Autodesk Inventor part; units mm, degrees
ref_plane "YZ Plane" through (0, 0, 0) normal (1, 0, 0) x (0, 1, 0)
ref_plane "XZ Plane" through (0, 0, 0) normal (0, 1, 0) x (-1, 0, 0)
ref_plane "XY Plane" through (0, 0, 0) normal (0, 0, 1) x (1, 0, 0)
sketch "Sketch1" plane through (0, 0, 0) normal (0, 0, 1) x (1, 0, 0)
  line L0 (-94, 50) -> (94, 50)
  line L1 (94, 50) -> (94, -50)
  line L2 (94, -50) -> (-94, -50)
  line L3 (-94, -50) -> (-94, 50)
  point P0 (0, 0)
  point P1 (0, 50)
  point P2 (94, 0)
  dimension "d2" = 100
  dimension "d3" = 188
extrude "Extrusion1" add sketch "Sketch1" along normal blind 6
sketch "Sketch5" plane through (0, 0, 6) normal (0, 0, 1) x (1, 0, 0)
  circle A0 centre (82, -43.9615) radius 1.7
  circle A1 centre (82, 43.9615) radius 1.7
  line L0 (82, -43.9615) -> (82, 43.9615) construction
  line L1 (94, -50) -> (94, 50)
  point P0 (0, 0)
  point P1 (82, 0)
  point P2 (94, 0)
  dimension "d27" = 3.4
  dimension "d28" = 12
  dimension "d29" = 87.923
extrude "Extrusion5" cut sketch "Sketch5" against normal through all
sketch "Sketch6" plane through (0, 0, 6) normal (0, 0, 1) x (1, 0, 0)
  line L0 (70, 25) -> (94, 25)
  line L1 (94, 25) -> (94, -25)
  line L2 (94, -25) -> (70, -25)
  line L3 (70, -25) -> (70, 25)
  line L4 (94, -50) -> (94, 50)
  point P0 (0, 0)
  point P1 (94, 0)
  dimension "d34" = 24
  dimension "d35" = 50
extrude "Extrusion6" cut sketch "Sketch6" against normal through all
fillet "Fillet2" radius 6 2 edges at (70, -25, 3) (70, 25, 3)
fillet "Fillet3" radius 3 6 edges at (94, -25, 3) (94, -50, 3) (94, 25, 3) (94, 50, 3) (-94, 50, 3) (-94, -50, 3)
sketch "Sketch9" plane through (0, 0, 6) normal (0, 0, 1) x (1, 0, 0)
  circle A0 centre (-82, 43.9615) radius 1.7
  circle A1 centre (-82, -43.9615) radius 1.7
  line L0 (-82, -43.9615) -> (-82, 43.9615) construction
  line L1 (-94, 47) -> (-94, -47)
  point P0 (0, 0)
  point P1 (-82, 0)
  point P2 (-94, 0)
  dimension "d47" = 87.923
  dimension "d48" = 12
  dimension "d49" = 3.4
extrude "Extrusion8" cut sketch "Sketch9" against normal through all
sketch "Sketch10" plane through (0, 0, 6) normal (0, 0, 1) x (1, 0, 0)
  line L0 (-94, 47) -> (-94, -47)
  line L1 (-94, -25) -> (-74, -25)
  line L2 (-74, -25) -> (-74, 25)
  line L3 (-74, 25) -> (-94, 25)
  line L4 (-94, 25) -> (-94, -25)
  point P0 (0, 0)
  point P1 (-94, 0)
  dimension "d52" = 50
  dimension "d53" = 20
extrude "Extrusion9" cut sketch "Sketch10" against normal through all
fillet "Fillet4" radius 6 4 edges at (-74, -25, 3) (-74, 25, 3) (-94, -25, 3) (-94, 25, 3)
chamfer "Chamfer5" distance 1 angle 45 48 edges at (0, -50, 6) (93.1213, -49.1213, 6) (94, -37.5, 6) (93.1213, -25.8787, 6) (83.5, -25, 6) (71.7574, -23.2426, 6) (70, 0, 6) (71.7574, 23.2426, 6) (83.5, 25, 6) (93.1213, 25.8787, 6) (94, 37.5, 6) (93.1213, 49.1213, 6) (0, 50, 6) (-93.1213, 49.1213, 6) (-94, 39, 6) (-92.2426, 26.7574, 6) (-84, 25, 6) (-75.7574, 23.2426, 6) (-74, 0, 6) (-75.7574, -23.2426, 6) (-84, -25, 6) (-92.2426, -26.7574, 6) (-94, -39, 6) (-93.1213, -49.1213, 6) (0, 50, 0) (-93.1213, 49.1213, 0) (-94, 39, 0) (-92.2426, 26.7574, 0) (-84, 25, 0) (-75.7574, 23.2426, 0) (-74, 0, 0) (-75.7574, -23.2426, 0) (-84, -25, 0) (-92.2426, -26.7574, 0) (-94, -39, 0) (-93.1213, -49.1213, 0) (0, -50, 0) (93.1213, -49.1213, 0) (94, -37.5, 0) (93.1213, -25.8787, 0) (83.5, -25, 0) (71.7574, -23.2426, 0) (70, 0, 0) (71.7574, 23.2426, 0) (83.5, 25, 0) (93.1213, 25.8787, 0) (94, 37.5, 0) (93.1213, 49.1213, 0)
properties part number "Cathode-Cover-Plate-bottom-side"
Here's how the part is built. I have some questions about the finished solid (model axes, mm). A direction names the side the tool comes from. Give positions to 0.01 mm unless a question says otherwise; leave off trailing zeros. Loops run counter-clockwise (first coordinate to the right, second up) from the corner with the lowest first, then second, coordinate; pieces in that order, holes last. Notation, with made-up numbers: M 65.5,35 L 87.5,35 A23 ccw 87.5,52 Z; hole C 5,89 d4. An arc over 180 degrees is marked long. Return JSON: item names as keys, results as strings.
Item 1: I'm going to push flat-ended pins straight in: pin 1 Ø3 at (y, z) = (18.5, 1) entering from +X; pin 2 Ø3 at (y, z) = (9.5, 4) entering from -X; pin 3 Ø2.5 at (x, y) = (-82, 43.96) entering from +Z; pin 4 Ø2 at (y, z) = (-3.5, 3) entering from +X. Where does each tip first touch, or does it pass through?
A:
{"pin 1": "stops at x = 70.08", "pin 2": "stops at x = -74", "pin 3": "passes through", "pin 4": "stops at x = 70"}
Item 2: Imagine slicing it at A-A on z = 3.5. List the corners of the cut face in (x, y) for me.
A:
{"outline": "M -94,-47 A3 ccw -91,-50 L 91,-50 A3 ccw 94,-47 L 94,-28 A3 ccw 91,-25 L 76,-25 A6 cw 70,-19 L 70,19 A6 cw 76,25 L 91,25 A3 ccw 94,28 L 94,47 A3 ccw 91,50 L -91,50 A3 ccw -94,47 L -94,31 A6 ccw -88,25 L -80,25 A6 cw -74,19 L -74,-19 A6 cw -80,-25 L -88,-25 A6 ccw -94,-31 Z; hole C -82,-43.96 d3.4; hole C -82,43.96 d3.4; hole C 82,-43.96 d3.4; hole C 82,43.96 d3.4"}
Item 3: On a 3-axis mill with a long thin cutter (end or side, diameter ignored), from which of +Z, -Z, +X, -X, +Y, -Y can I reach the whole of each face in a straight line? I mean faces 4 (the conical face through (-75.683, 23.413, 0.826)), 5 (the cylindrical face through (71.804, -23.289, 2.972)), 6 (the conical face through (71.683, -23.413, 0.826)), 7 (the cylindrical face through (-92.289, -26.804, 2.972)). Say none if no direction works.
A:
{"face 4": "-Z, -X", "face 5": "+Z, -Z, +X", "face 6": "-Z, +X", "face 7": "+Z, -Z, -X"}
Item 4: Thinking about a two-plate mould opening in Y: for faces 1 (the conical face through (-75.587, -23.317, 0.826)), 2 (the flat face through (-1, 50, 3)), 3 (the flat face through (-1, 1, 6)), which applies, released by +Y, released by -Y, zero draft, split by the parting line, or undercut?
A:
{"face 1": "undercut", "face 2": "released by +Y", "face 3": "zero draft"}
Item 5: Please list where these lines run through material, in increasing order: line 1 (Y direction, x = 82, z = 1.9); line 2 (X direction, y = 43, z = 4.6); line 3 (X direction, y = 44, z = 1.8).
A:
{"line 1": "y = -50 to -45.66, -42.26 to -25, 25 to 42.26, 45.66 to 50", "line 2": "x = -94 to -83.4, -80.6 to 80.6, 83.4 to 94", "line 3": "x = -94 to -83.7, -80.3 to 80.3, 83.7 to 94"}
